Autodesk Inventor part; units mm, degrees
ref_plane "YZ Plane" through (0, 0, 0) normal (1, 0, 0) x (0, 1, 0)
ref_plane "XZ Plane" through (0, 0, 0) normal (0, 1, 0) x (-1, 0, 0)
ref_plane "XY Plane" through (0, 0, 0) normal (0, 0, 1) x (1, 0, 0)
sketch "Esquisse1" plane through (0, 0, 0) normal (0, 1, 0) x (-1, 0, 0)
  line L0 (-9.5, -40) -> (-12.5, -40)
  line L1 (-12.5, -40) -> (-12.5, 10)
  line L2 (-12.5, 10) -> (-9.5, 10)
  line L3 (-9.5, 10) -> (-9.5, -40)
  line L4 (9.5, 40) -> (12.5, 40)
  line L5 (12.5, 40) -> (12.5, -40)
  line L6 (12.5, -40) -> (9.5, -40)
  line L7 (9.5, -40) -> (9.5, 40)
  line L8 (-9.5, -20) -> (9.5, -20)
  line L9 (9.5, -20) -> (9.5, -17)
  line L10 (9.5, -17) -> (-9.5, -17)
  line L11 (-9.5, -17) -> (-9.5, -20)
  point P0 (0, 0)
  dimension "d0" = 3
  dimension "d1" = 3
  dimension "d2" = 3
  dimension "d4" = 25
  dimension "d5" = 80
  dimension "d6" = 40
  dimension "d7" = 12.5
  dimension "d11" = 57
  dimension "d12" = 30
extrude "Extrusion1" add sketch "Esquisse1" along normal blind 30
fillet "Congé1" radius 14 4 edges at (11, 30, -40) (-11, 30, -40) (11, 0, -40) (-11, 0, -40)
sketch "Esquisse2" plane through (-12.5, 0, 40) normal (-1, 0, 0) x (0, 0, 1)
  line L0 (0, 0) -> (0, 30)
  line L1 (-80, 14) -> (-80, 16)
  line L2 (-49, 25.5) -> (-7, 25.5)
  line L3 (-7, 25.5) -> (-7, 4.5)
  line L4 (-7, 4.5) -> (-49, 4.5)
  line L5 (-49, 4.5) -> (-49, 25.5)
  line L6 (0, 15) -> (-80, 15) construction
  line L7 (-7, 25.5) -> (0, 25.5) construction
  line L8 (0, 25.5) -> (0, 4.5) construction
  line L9 (0, 4.5) -> (-7, 4.5) construction
  line L10 (-7, 4.5) -> (-7, 25.5) construction
  line L11 (-49, 25.5) -> (-56, 25.5) construction
  line L12 (-56, 25.5) -> (-56, 4.5) construction
  line L13 (-56, 4.5) -> (-49, 4.5) construction
  line L14 (-49, 4.5) -> (-49, 25.5) construction
  circle A0 centre (-52.2, 20.6) radius 2.5
  circle A1 centre (-52.2, 9.4) radius 2.5
  circle A2 centre (-3.8, 9.4) radius 2.5
  circle A3 centre (-3.8, 20.6) radius 2.5
  point P0 (-40, 0)
  dimension "d16" = 21
  dimension "d17" = 10.5
  dimension "d18" = 7
  dimension "d19" = 42
  dimension "d20" = 7
  dimension "d21" = 7
  dimension "d22" = 5
  dimension "d23" = 4.9
  dimension "d24" = 3.8
  dimension "d25" = 5
  dimension "d26" = 5
  dimension "d27" = 5
  dimension "d28" = 3.8
  dimension "d29" = 4.9
  dimension "d30" = 3.8
  dimension "d31" = 4.9
  dimension "d32" = 3.8
  dimension "d33" = 4.9
extrude "Extrusion2" cut sketch "Esquisse2" against normal through all
fillet "Congé2" radius 5 1 edges at (-11, 0, 40)
fillet "Congé3" radius 5 1 edges at (-11, 30, 40)
fillet "Congé4" radius 5 1 edges at (11, 0, 10)
fillet "Congé5" radius 5 1 edges at (11, 30, 10)
equation "\"d17\" = 0.5 * d16"
equation "\"d21\" = d20"
equation "\"d25\" = d22"
equation "\"d26\" = d22"
equation "\"d27\" = d22"
equation "\"d28\" = d24"
equation "\"d29\" = d23"
equation "\"d30\" = d24"
equation "\"d31\" = d23"
equation "\"d32\" = d24"
equation "\"d33\" = d23"
properties part number "new_leg_2"
CAD build for the part. Positions are in the model's coordinates, mm. A direction names the side the tool comes from. Give positions to 0.01 mm unless a question says otherwise; leave off trailing zeros. Write each loop counter-clockwise with the first axis right and the second up, starting at its lowest first coordinate (ties: lowest second). Pieces come first, ordered by that corner, then holes. Notation, with made-up numbers: (-10, 24.25) -> (10, 24.25) arc R13 ccw to (10, 44.25) -> close; hole circle Ø4 at (52, -7.75). An arc over 180 degrees is marked (long way). Write each question's results on one line, items separated by ' | '.
1. Which spindle directions (+Z, -Z, +X, -X, +Y, -Y) get a long thin tool onto all of the face, cutting with end or side? Do faces 5 (the flat face through (-11, 15, -9)), 6 (the flat face through (11, 25.5, 0)), 7 (the flat face through (-9.5, 15, -28)), 8 (the flat face through (9.5, 14.8, -9.3)). Say none if no direction does.
Geometry check:
face 5: +X, -X | face 6: +Z, +X, -X | face 7: -Z, +Y, -Y | face 8: +Z, +Y, -Y
2. Wall check: probe 1 along X at (y, z) = (26.75, -9.5); probe 2 along Y at (x, z) = (-11.5, 36.2); probe 3 along Z at (x, y) = (-10.25, 15.75). Give the ranges that are in metal, low to high. Write a range as [from, to].
Geometry check:
probe 1: [-12.5, -9.5], [9.5, 12.5] | probe 2: [0.15, 6.9], [11.9, 18.1], [23.1, 29.85] | probe 3: [-40, -9], [33, 40]
3. Cut at C-C, the plane z = 36.2. Write the cut outline in (x, y).
Geometry check:
outline: (-12.5, 0.15) -> (-9.5, 0.15) -> (-9.5, 6.9) -> (-12.5, 6.9) -> close; (-12.5, 11.9) -> (-9.5, 11.9) -> (-9.5, 18.1) -> (-12.5, 18.1) -> close; (-12.5, 23.1) -> (-9.5, 23.1) -> (-9.5, 29.85) -> (-12.5, 29.85) -> close
4. Two-plate mould, pull along Y, no slides. Class faces 1 (the flat face through (9.5, 15, -30)), 2 (the cylindrical face through (11.021, 28.742, 8.341)), 3 (the flat face through (-11, 4.5, 12)), 4 (the cylindrical face through (10.98, 18.16, -12.74)): pulls with the +Y half, pulls with the -Y half, needs draft (parallel to the pull), parting line crosses it, or undercut.
Geometry check:
face 1: needs draft | face 2: pulls with the +Y half | face 3: undercut | face 4: undercut
5. Cut at B-B, the plane x = -10.5. Write the cut outline in (y, z).
Geometry check:
outline: (0, -26) arc R14 ccw to (14, -40) -> (16, -40) arc R14 ccw to (30, -26) -> (30, 35) arc R5 ccw to (25, 40) -> (5, 40) arc R5 ccw to (0, 35) -> close; hole (4.5, -9) -> (25.5, -9) -> (25.5, 33) -> (4.5, 33) -> close; hole circle Ø5 at (9.4, -12.2); hole circle Ø5 at (9.4, 36.2); hole circle Ø5 at (20.6, -12.2); hole circle Ø5 at (20.6, 36.2)
6. Cut at D-D, the plane y = 9.4. Write the cut outline in (x, z).
Geometry check:
outline: (-12.5, -39.22) -> (-9.5, -39.22) -> (-9.5, -20) -> (9.5, -20) -> (9.5, -39.22) -> (12.5, -39.22) -> (12.5, -14.7) -> (9.5, -14.7) -> (9.5, -17) -> (-9.5, -17) -> (-9.5, -14.7) -> (-12.5, -14.7) -> close; (-12.5, -9.7) -> (-9.5, -9.7) -> (-9.5, -9) -> (-12.5, -9) -> close; (-12.5, 33) -> (-9.5, 33) -> (-9.5, 33.7) -> (-12.5, 33.7) -> close; (-12.5, 38.7) -> (-9.5, 38.7) -> (-9.5, 40) -> (-12.5, 40) -> close; (9.5, -9.7) -> (12.5, -9.7) -> (12.5, -9) -> (9.5, -9) -> close
7. Cut at A-A, the plane z = -12.2. Write the cut outline in (x, y), then the cut area to 3 significant figures.
Geometry check:
outline: (-12.5, 0) -> (-9.5, 0) -> (-9.5, 6.9) -> (-12.5, 6.9) -> close; (-12.5, 11.9) -> (-9.5, 11.9) -> (-9.5, 18.1) -> (-12.5, 18.1) -> close; (-12.5, 23.1) -> (-9.5, 23.1) -> (-9.5, 30) -> (-12.5, 30) -> close; (9.5, 0) -> (12.5, 0) -> (12.5, 6.9) -> (9.5, 6.9) -> close; (9.5, 11.9) -> (12.5, 11.9) -> (12.5, 18.1) -> (9.5, 18.1) -> close; (9.5, 23.1) -> (12.5, 23.1) -> (12.5, 30) -> (9.5, 30) -> close | area: 120 mm²
8. Drop flat-ended pins along their axis: P1, Ø5, axis at x = 0, y = 9, coming from the -Z side; P2, Ø15, axis at y = 9.5, z = 22, coming from the +X side; P3, Ø4, axis at x = 3.5, y = 19, coming from the +Z side. Give the stop position or say it passes through.
Geometry check:
P1: z = -20 | P2: x = -9.5 | P3: z = -17
